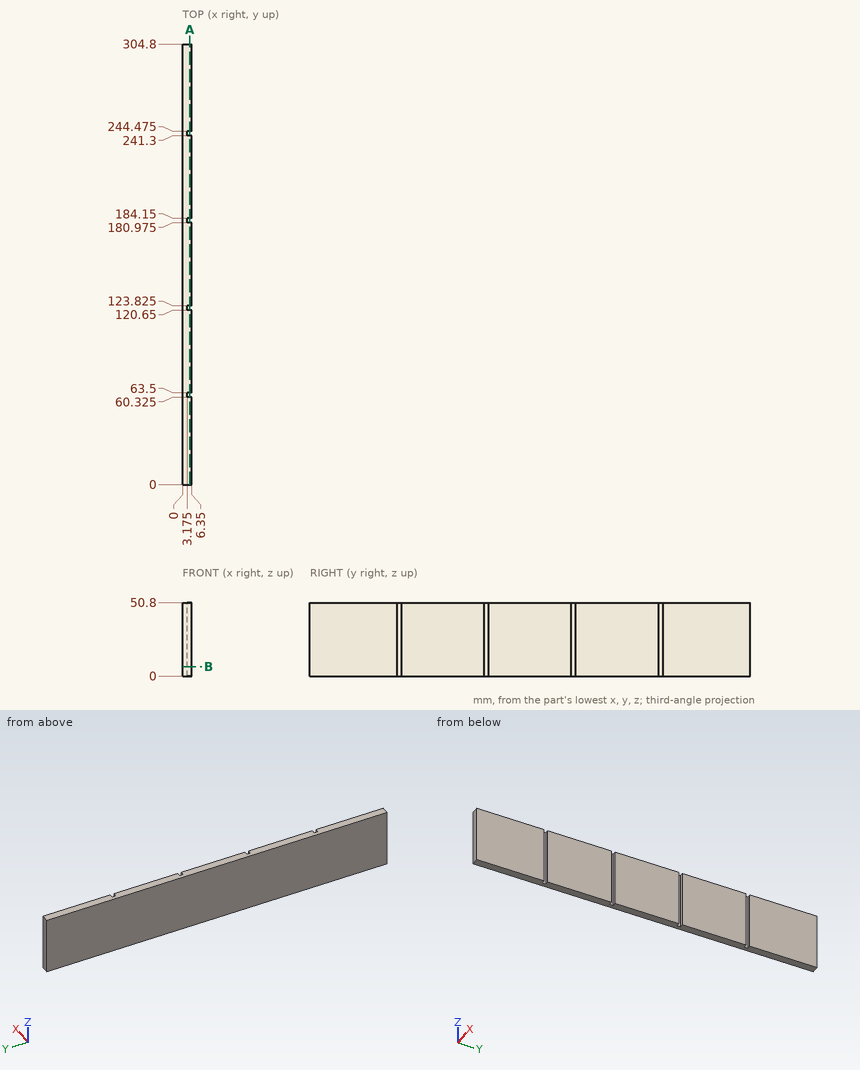
Geometry check sheet. Reference: drawing and pictorial views, mm from the part's lowest x, y, z. Round coordinates to 2 decimals unless told otherwise and drop trailing zeros. Order: outer loops, then holes, each group sorted by start corner. A loop starts at its lowest first (then second) coordinate and runs counter-clockwise, first axis right, second up. Notation, with made-up numbers: (71.25, -24) - (109.25, -24) arc R17 cw to (109.25, -3) - close; hole circle Ø4 at (15.5, 33.5). An arc over 180 degrees is marked (long way). One line per question, with ' | ' between items. Start each with the question number.
(1) Sectioned sample at A-A on x = 5. Record the cut outline in (y, z) (3 decimals).
(2) Sectioned sample at B-B on z = 6.5. Record the cut outline in (x, y) (3 decimals), and give its area (3 significant figures).
(3) Thickness scan on L1, parallel to Y at x = 3.5, z = 33 (3 decimals). Record the ranges inside material, lowest first. Write a range as [from, to].
(4) Depth check by flat-ended pin: pin 1 Ø2.5 at (x, z) = (4.5, 35.5) entering from -Y; pin 2 Ø1 at (y, z) = (242.5, 13) entering from +X (3 decimals). Enter the tip coordinate at first touch or a pass-through.
Conclusion:
1) outline: (0, 0) - (60.325, 0) - (60.325, 50.8) - (0, 50.8) - close; (63.5, 0) - (120.65, 0) - (120.65, 50.8) - (63.5, 50.8) - close; (123.825, 0) - (180.975, 0) - (180.975, 50.8) - (123.825, 50.8) - close; (184.15, 0) - (241.3, 0) - (241.3, 50.8) - (184.15, 50.8) - close; (244.475, 0) - (304.8, 0) - (304.8, 50.8) - (244.475, 50.8) - close
2) outline: (0, 0) - (6.35, 0) - (6.35, 60.325) - (3.175, 60.325) - (3.175, 63.5) - (6.35, 63.5) - (6.35, 120.65) - (3.175, 120.65) - (3.175, 123.825) - (6.35, 123.825) - (6.35, 180.975) - (3.175, 180.975) - (3.175, 184.15) - (6.35, 184.15) - (6.35, 241.3) - (3.175, 241.3) - (3.175, 244.475) - (6.35, 244.475) - (6.35, 304.8) - (0, 304.8) - close | area: 1,900 mm2
3) L1: y = [0, 60.325], [63.5, 120.65], [123.825, 180.975], [184.15, 241.3], [244.475, 304.8]
4) pin 1: stops at y = 0 | pin 2: stops at x = 3.175
